Part model, mm, in its own coordinate system. A direction names the side the tool comes from. Round coordinates to 2 decimals unless told otherwise and drop trailing zeros. Loops run counter-clockwise (first coordinate to the right, second up) from the corner with the lowest first, then second, coordinate; pieces in that order, holes last. Notation, with made-up numbers: M -26,24.25 L 21,24.25 A18 ccw 21,36.25 Z; hole C 79,67.25 d3. An arc over 180 degrees is marked long. Put each result on its own line as item: value. Start each with the question number.
```python
from build123d import *

# Parameters (mm, degrees)
DODANIE_WYCI_GNI_CIE1_DEPTH = 45
ZAOKR_GLENIE2_R             = 0.1


with BuildPart() as part:
    # Szkic1 → Dodanie-wyciągnięcie1 (new body)
    with BuildSketch(Plane(origin=(0, 0, 0), x_dir=(1, 0, 0), z_dir=(0, 1, 0))):
        Polygon((0, 0), (15, 0), (15, 1.2), (1.2, 1.2), (1.2, 15), (0, 15), align=None)
    extrude(amount=DODANIE_WYCI_GNI_CIE1_DEPTH)

    # Zaokrąglenie2
    zaokr_glenie2_edges = [part.edges().sort_by_distance(p)[0] for p in [
        (0, 22.5, -15),
        (1.2, 22.5, -15),
        (1.2, 22.5, -1.2),
        (15, 22.5, -1.2),
        (15, 22.5, 0),
        (0, 22.5, 0),
    ]]
    fillet(zaokr_glenie2_edges, radius=ZAOKR_GLENIE2_R)


solid = part.part
```
1. Cut at A-A, the plane y = 12. Give the cut face in (x, z), and give its area (3 significant figures).
2. Which spindle directions (+Z, -Z, +X, -X, +Y, -Y) get a long thin tool onto all of the face, cutting with end or side? Do faces 1 (the flat face through (0.6, 22.2, -15)), 2 (the flat face through (1.2, 22, -8)). Say none if no direction does.
3. Cut at B-B, the plane z = -5. Give the cut face in (x, y), and give its area (3 significant figures).
4. Cut at C-C, the plane x = 14. Give the cut face in (y, z), and give its area (3 significant figures).
5. Wall check: L1, parallel to X at y = 2, z = -4.25; L2, parallel to Z at x = 10, y = 16. Give the ranges that are in metal, low to high.
6. Drop flat-ended pins along their axis: pin 1 (2 mm diameter, centred on x = 3.5, y = 14.5, fed in from -Z); pin 2 (8 mm diameter, centred on y = 9, z = -8.5, fed in from +X); pin 3 (1 mm diameter, centred on x = 3.5, z = -8.5, fed in from +Y). Give the stop position or say it passes through.
Results list:
1. outline: M 0,-14.9 A0.1 ccw 0.1,-15 L 1.1,-15 A0.1 ccw 1.2,-14.9 L 1.2,-1.3 A0.1 cw 1.3,-1.2 L 14.9,-1.2 A0.1 ccw 15,-1.1 L 15,-0.1 A0.1 ccw 14.9,0 L 0.1,0 A0.1 ccw 0,-0.1 Z
1. area: 34.6 mm^2
2. face 1: -Z, +X, -X, +Y, -Y
2. face 2: -Z, +X, +Y, -Y
3. outline: M 0,0 L 1.2,0 L 1.2,45 L 0,45 Z
3. area: 54.0 mm^2
4. outline: M 0,-1.2 L 45,-1.2 L 45,0 L 0,0 Z
4. area: 54.0 mm^2
5. L1: x = 0 to 1.2
5. L2: z = -1.2 to 0
6. pin 1: stops at z = -1.2
6. pin 2: stops at x = 1.2
6. pin 3: passes through
